```python
from build123d import *

# Parameters (mm, degrees)
SKETCH_1_R      = 2
SKETCH_1_R_2    = 8.75
SKETCH_1_R_3    = 1.5
SKETCH_1_W      = 2.2
SKETCH_1_H      = 4.2
SKETCH_1_W_2    = 4.2
EXTRUDE_1_DEPTH = 2


with BuildPart() as part:
    # 草图1 → 凸台-拉伸1 (new body)
    with BuildSketch(Plane(origin=(0, 0, 0), x_dir=(0, 0, -1), z_dir=(1, 0, 0))):
        with BuildLine():
            Line((21.45, -20.5), (37.442185592, -20.5))
            ThreePointArc((37.442185592, -20.5), (48.468724148, 0), (37.442185592, 20.5))
            Line((37.442185592, 20.5), (21.45, 20.5))
            Line((21.45, 20.5), (5.457814408, 20.5))
            ThreePointArc((5.457814408, 20.5), (-4.55, 0), (5.457814408, -20.5))
            Line((5.457814408, -20.5), (21.45, -20.5))
        make_face()
        with Locations((21.45, 15)):
            Circle(SKETCH_1_R, mode=Mode.SUBTRACT)
        with Locations((21.45, -15)):
            Circle(SKETCH_1_R, mode=Mode.SUBTRACT)
        with Locations((21.45, 0)):
            Circle(SKETCH_1_R_2, mode=Mode.SUBTRACT)
        Circle(SKETCH_1_R_3, mode=Mode.SUBTRACT)
        with Locations((42.9, 0)):
            Circle(SKETCH_1_R_3, mode=Mode.SUBTRACT)
        with Locations((0, 6)):
            Rectangle(SKETCH_1_W, SKETCH_1_H, mode=Mode.SUBTRACT)
        with Locations((0, -6)):
            Rectangle(SKETCH_1_W, SKETCH_1_H, mode=Mode.SUBTRACT)
        with Locations((42.9, 6)):
            Rectangle(SKETCH_1_W_2, SKETCH_1_H, mode=Mode.SUBTRACT)
        with Locations((42.9, -6)):
            Rectangle(SKETCH_1_W_2, SKETCH_1_H, mode=Mode.SUBTRACT)
    extrude(amount=EXTRUDE_1_DEPTH)


solid = part.part
```
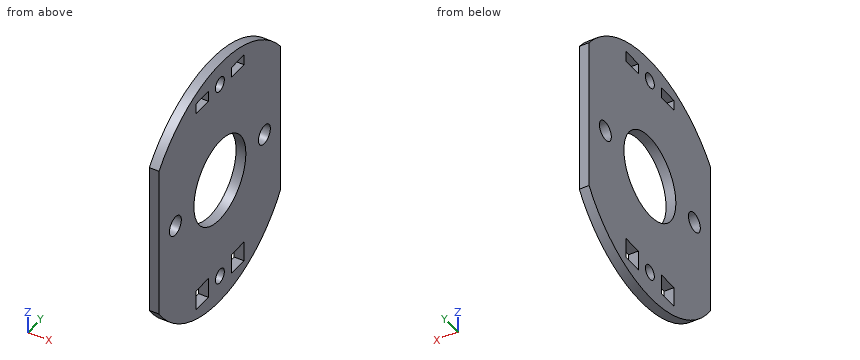
Input: part model. Units: mm. Frame: model coordinates. Give positions to 0.01 mm unless a question says otherwise; leave off trailing zeros. Order: outer loops, then holes, each group sorted by start corner. A loop starts at its lowest first (then second) coordinate and runs counter-clockwise, first axis right, second up.
1. Cut plane B-B (y = 0). Return loops of the section in (x, z), and give its area (3 significant figures).
Computed:
outline: (0, -48.47) - (2, -48.47) - (2, -44.4) - (0, -44.4) - close; (0, -41.4) - (2, -41.4) - (2, -30.2) - (0, -30.2) - close; (0, -12.7) - (2, -12.7) - (2, -1.5) - (0, -1.5) - close; (0, 1.5) - (2, 1.5) - (2, 4.55) - (0, 4.55) - close
area: 59.0 mm2
2. Line query: probe 1 along Y at (x, z) = (1.4, -21.45); probe 2 along Y at (x, z) = (0.75, -44); probe 3 along Z at (x, y) = (0.95, 5). Output: solid intervals per line, ascending.
Computed:
probe 1: y = -20.5 to -17, -13 to -8.75, 8.75 to 13, 17 to 20.5
probe 2: y = -14.13 to -8.1, -3.9 to -1.02, 1.02 to 3.9, 8.1 to 14.13
probe 3: z = -47.95 to -45, -40.8 to -28.63, -14.27 to -1.1, 1.1 to 4.06
3. Pin query (flat end, axial travel): pin 1 Ø3.5 at (y, z) = (15, -21.45) entering from -X; pin 2 Ø0.6 at (x, z) = (1, -0.5) entering from +Y; pin 3 Ø1 at (x, z) = (1, -42.5) entering from -Y; pin 4 Ø1 at (x, y) = (1.5, 5.5) entering from -Z. Return the tip coordinate at first contact, or that it passes through.
Computed:
pin 1: passes through
pin 2: stops at y = 15.8
pin 3: stops at y = -16.61
pin 4: stops at z = -47.95
4. Cut plane D-D (y = 15). Return loops of the section in (x, z), and give its area (3 significant figures).
Computed:
outline: (0, -43.36) - (2, -43.36) - (2, -23.45) - (0, -23.45) - close; (0, -19.45) - (2, -19.45) - (2, -0.21) - (0, -0.21) - close
area: 78.3 mm2
5. Cut plane C-C (x = 1). State how many separate pieces and enclosed holes the cut face has, and give its area (3 significant figures).
Computed:
separate pieces: 1
enclosed holes: 9
area: 1,580 mm2
6. Cut plane A-A (z = -21.45). Return loops of the section in (x, y).
Computed:
outline: (0, -20.5) - (2, -20.5) - (2, -17) - (0, -17) - close; (0, -13) - (2, -13) - (2, -8.75) - (0, -8.75) - close; (0, 8.75) - (2, 8.75) - (2, 13) - (0, 13) - close; (0, 17) - (2, 17) - (2, 20.5) - (0, 20.5) - close
